For this review, take the finished solid that the model builds, in its own axes (mm). Face numbers are marked on the shaded views. A direction names the side the tool comes from. Round coordinates to 2 decimals unless told otherwise and drop trailing zeros. Write each loop counter-clockwise with the first axis right and the second up, starting at its lowest first coordinate (ties: lowest second). Pieces come first, ordered by that corner, then holes.
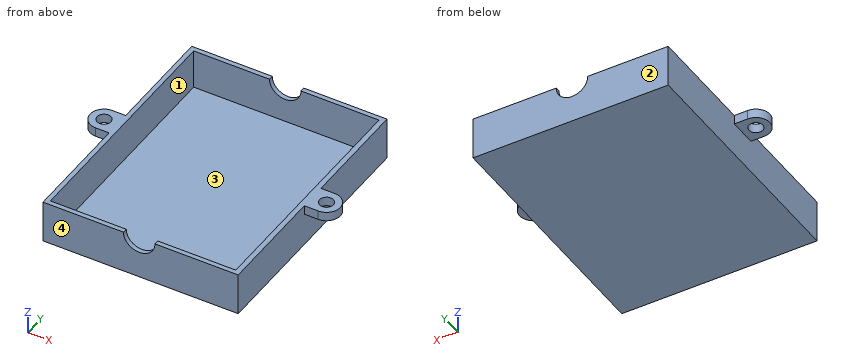
from build123d import *

# Parameters (mm, degrees)
SKETCH2_W                = 200
SKETCH2_H                = 258.87959476
BOSS_EXTRUDE1_DEPTH      = 3
SKETCH6_W                = 200
SKETCH6_H                = 258.87959476
BOSS_EXTRUDE2_DEPTH      = 43
BOSS_EXTRUDE2_DEPTH_BACK = 3
SKETCH7_R                = 17
CUT_EXTRUDE1_DEPTH       = 1
CUT_EXTRUDE1_DEPTH_BACK  = 269.87959476
SKETCH9_R                = 7.5
BOSS_EXTRUDE3_DEPTH      = 10


with BuildPart() as part:
    # Sketch2 → Boss-Extrude1 (new body)
    with BuildSketch(Plane(origin=(0, 0, 0), x_dir=(-1, 0, 0), z_dir=(0, 0, 1))):
        with Locations((-1.649083583, 6.704740248)):
            Rectangle(SKETCH2_W, SKETCH2_H)
    extrude(amount=BOSS_EXTRUDE1_DEPTH)

    # Sketch6 → Boss-Extrude2 (add, two sides)
    with BuildSketch(Plane.XY.offset(3)) as boss_extrude2_sk:
        Polygon((-98.350916417, 127.735057132), (-103.350916417, 127.735057132), (-103.350916417, 122.735057132), (-103.350916417, -141.144537628), (107.252666614, -141.144537628), (107.252666614, 127.735057132), align=None)
        with Locations((1.649083583, -6.704740248)):
            Rectangle(SKETCH6_W, SKETCH6_H, mode=Mode.SUBTRACT)
    extrude(amount=BOSS_EXTRUDE2_DEPTH)
    extrude(boss_extrude2_sk.sketch, amount=-BOSS_EXTRUDE2_DEPTH_BACK)

    # Sketch7 → Cut-Extrude1 (cut, two sides)
    with BuildSketch(Plane.XZ.offset(141.144537628)) as cut_extrude1_sk:
        with Locations((0.452666614, 46)):
            Circle(SKETCH7_R)
    extrude(amount=CUT_EXTRUDE1_DEPTH, mode=Mode.SUBTRACT)
    extrude(cut_extrude1_sk.sketch, amount=-CUT_EXTRUDE1_DEPTH_BACK, mode=Mode.SUBTRACT)

    # Sketch9 → Boss-Extrude3 (add)
    with BuildSketch(Plane.XY.offset(46)):
        with BuildLine():
            Line((107.252666614, 8.295259752), (107.252666614, -6.704740248))
            Line((107.252666614, -6.704740248), (107.252666614, -21.704740248))
            Line((107.252666614, -21.704740248), (122.252666614, -21.704740248))
            ThreePointArc((122.252666614, -21.704740248), (137.252666614, -6.704740248), (122.252666614, 8.295259752))
            Line((122.252666614, 8.295259752), (107.252666614, 8.295259752))
        make_face()
        with Locations((122.252666614, -6.704740248)):
            Circle(SKETCH9_R, mode=Mode.SUBTRACT)
        with BuildLine():
            Line((-102.747333386, -21.704740248), (-102.747333386, -6.704740248))
            Line((-102.747333386, -6.704740248), (-102.747333386, 8.295259752))
            Line((-102.747333386, 8.295259752), (-117.747333386, 8.295259752))
            ThreePointArc((-117.747333386, 8.295259752), (-132.747333386, -6.704740248), (-117.747333386, -21.704740248))
            Line((-117.747333386, -21.704740248), (-102.747333386, -21.704740248))
        make_face()
        with Locations((-117.747333386, -6.704740248)):
            Circle(SKETCH9_R, mode=Mode.SUBTRACT)
    extrude(amount=-BOSS_EXTRUDE3_DEPTH)


solid = part.part
(1) We need section B-B, the plane x = 51.5. Give the boundary of the cut face in (y, z), and give its area (3 significant figures).
Geometry check:
outline: (-141.14, 0) - (127.74, 0) - (127.74, 46) - (122.74, 46) - (122.74, 3) - (-136.14, 3) - (-136.14, 46) - (-141.14, 46) - close
area: 1,240 mm2
(2) Mouldability with a two-part tool opening along X and no side actions: class the marked faces 3 and 4 as pulls with the +X half, pulls with the -X half, needs draft (parallel to the pull), parting line crosses it, or undercut.
Geometry check:
face 3: undercut
face 4: needs draft
(3) For pin 1 Ø15 at (x, y) = (116.5, -4) entering from -Z; pin 2 Ø13 at (y, z) = (-61.5, 34) entering from -X; pin 3 Ø12 at (y, z) = (17, 34.5) entering from +X; pin 4 Ø6 at (x, y) = (-30, -48.5) entering from -Z, all flat-tipped, find the tip position at first contact; note any pin that passes through.
Geometry check:
pin 1: stops at z = 36
pin 2: stops at x = -103.35
pin 3: stops at x = 107.25
pin 4: stops at z = 0
(4) For line 1 along X through (y, z) = (-129, 22); line 2 along Y through (x, z) = (38, 13.5); line 3 along Z through (x, y) = (43.5, -95), list the stretches that pass through material, from the lowest coordinate up.
Geometry check:
line 1: x = -103.35 to -98.35, 101.65 to 107.25
line 2: y = -141.14 to -136.14, 122.74 to 127.74
line 3: z = 0 to 3
(5) We need section C-C, the plane y = -30.5. Give the boundary of the cut face in (x, z), and give its area (3 significant figures).
Geometry check:
outline: (-103.35, 0) - (107.25, 0) - (107.25, 46) - (101.65, 46) - (101.65, 3) - (-98.35, 3) - (-98.35, 46) - (-103.35, 46) - close
area: 1,090 mm2
(6) For the marked faces 1 and 2, list the 3-axis set-ups (+Z, -Z, +X, -X, +Y, -Y) from which the entire face can be reached by the end or side of a thin tool; tool diameter is ignored.
Geometry check:
face 1: +Z
face 2: +Z, -Z, +X, -X, +Y
(7) We need section A-A, the plane z = 11. Give the boundary of the cut face in (x, y), and give its area (3 significant figures).
Geometry check:
outline: (-103.35, -141.14) - (107.25, -141.14) - (107.25, 127.74) - (-103.35, 127.74) - close; hole (-98.35, -136.14) - (101.65, -136.14) - (101.65, 122.74) - (-98.35, 122.74) - close
area: 4,850 mm2
